```python
from build123d import *

# Parameters (mm, degrees)
SKETCH1_W                 = 14.859
SKETCH1_H                 = 205.105
BOSS_EXTRUDE1_DEPTH       = 9.398
SKETCH2_W                 = 6.35
SKETCH2_H                 = 13.335
CUT_EXTRUDE1_DEPTH        = 206.591740717
F_5_CLEARANCE_HOLE1_D     = 3.556
F_5_CLEARANCE_HOLE1_DEPTH = 1.524
F_5_CLEARANCE_HOLE2_D     = 3.556
F_5_CLEARANCE_HOLE2_DEPTH = 14.859
F_5_CLEARANCE_HOLE3_D     = 3.556
F_5_CLEARANCE_HOLE3_DEPTH = 9.398
FILLET1_R                 = 0.635


with BuildPart() as part:
    # Sketch1 → Boss-Extrude1 (new body)
    with BuildSketch(Plane(origin=(4.699, 0, 0), x_dir=(0, 0, -1), z_dir=(1, 0, 0))):
        with Locations((5.9055, 102.5525)):
            Rectangle(SKETCH1_W, SKETCH1_H)
    extrude(amount=-BOSS_EXTRUDE1_DEPTH)

    # Sketch2 → Cut-Extrude1 (cut, through all)
    with BuildSketch(Plane.XZ):
        with Locations((0, -6.6675)):
            Rectangle(SKETCH2_W, SKETCH2_H)
    extrude(amount=-CUT_EXTRUDE1_DEPTH, mode=Mode.SUBTRACT)

    # #5 Clearance Hole1
    with Locations(Plane(origin=(-3.175, 0, 0), x_dir=(0, 0, -1), z_dir=(1, 0, 0))):
        with Locations((8.5725, 190.5635), (8.5725, 200.3425), (8.5725, 180.7845), (8.5725, 171.0055), (8.5725, 161.2265), (8.5725, 151.4475), (8.5725, 141.6685), (8.5725, 131.8895), (8.5725, 122.1105), (8.5725, 112.3315), (8.5725, 102.5525), (8.5725, 92.7735), (8.5725, 82.9945), (8.5725, 73.2155), (8.5725, 63.4365), (8.5725, 53.6575), (8.5725, 43.8785), (8.5725, 34.0995), (8.5725, 24.3205), (8.5725, 14.5415), (8.5725, 4.7625)):
            Hole(F_5_CLEARANCE_HOLE1_D / 2, depth=F_5_CLEARANCE_HOLE1_DEPTH)

    # #5 Clearance Hole2
    with Locations(Plane.XY.offset(1.524)):
        with Locations((0, 190.5635), (0, 200.3425), (0, 180.7845), (0, 171.0055), (0, 161.2265), (0, 151.4475), (0, 141.6685), (0, 131.8895), (0, 122.1105), (0, 112.3315), (0, 102.5525), (0, 92.7735), (0, 82.9945), (0, 73.2155), (0, 63.4365), (0, 53.6575), (0, 43.8785), (0, 34.0995), (0, 24.3205), (0, 14.5415), (0, 4.7625)):
            Hole(F_5_CLEARANCE_HOLE2_D / 2, depth=F_5_CLEARANCE_HOLE2_DEPTH)

    # #5 Clearance Hole3
    with Locations(Plane(origin=(4.699, 0, 0), x_dir=(0, 0, -1), z_dir=(1, 0, 0))):
        with Locations((8.5725, 190.5635), (8.5725, 200.3425), (8.5725, 180.7845), (8.5725, 171.0055), (8.5725, 161.2265), (8.5725, 151.4475), (8.5725, 141.6685), (8.5725, 131.8895), (8.5725, 122.1105), (8.5725, 112.3315), (8.5725, 102.5525), (8.5725, 92.7735), (8.5725, 82.9945), (8.5725, 73.2155), (8.5725, 63.4365), (8.5725, 53.6575), (8.5725, 43.8785), (8.5725, 34.0995), (8.5725, 24.3205), (8.5725, 14.5415), (8.5725, 4.7625)):
            Hole(F_5_CLEARANCE_HOLE3_D / 2, depth=F_5_CLEARANCE_HOLE3_DEPTH)

    # Fillet1
    fillet1_edges = [part.edges().sort_by_distance(p)[0] for p in [
        (3.937, 0, -13.335),
        (3.937, 205.105, -13.335),
        (-3.937, 205.105, -13.335),
        (-3.937, 0, -13.335),
    ]]
    fillet(fillet1_edges, radius=FILLET1_R)


solid = part.part
```
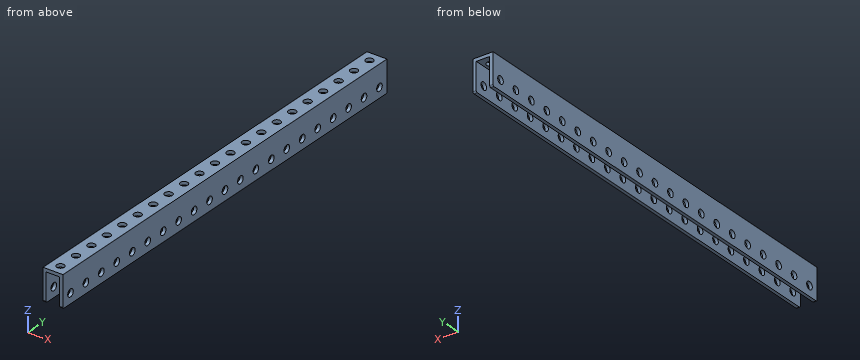
Geometry check sheet. Reference: the model listing, model coordinates, mm. Give positions to 0.01 mm unless a question says otherwise; leave off trailing zeros. Use one line per item in the form item = value.
Item 1: Depth check by flat-ended pin: pin 1 Ø4 at (x, y) = (0, 43.88) entering from -Z; pin 2 Ø3 at (y, z) = (63.44, -8.57) entering from -X. Enter the tip coordinate at first touch or a pass-through.
Results list:
pin_1 = 0
pin_2 = through
Item 2: Sectioned sample at A-A on x = 0. Count the separate pieces of the cut face and the enclosed holes in it, plus the area to 3 significant figures.
Results list:
separate_pieces = 22
enclosed_holes = 0
area = 199 mm2
Item 3: Scan lines: line 1 (X direction, y = 132, z = -0.5) (3 decimals); line 2 (Z direction, x = 3.5, y = 190.5) (3 decimals); line 3 (X direction, y = 73.5, z = 0.5). Record each from-to range of solid material in increasing order.
Results list:
line_1 = -4.699 to -3.175, 3.175 to 4.699
line_2 = -13.335 to -10.349, -6.796 to 1.524
line_3 = -4.7 to -1.76, 1.76 to 4.7
